Here's how the part is built. I have some questions about the finished solid (model axes, mm). Face numbers are marked on the shaded views. A direction names the side the tool comes from. Coordinates: 2 decimals unless noted, no trailing zeros. Write each loop counter-clockwise with the first axis right and the second up, starting at its lowest first coordinate (ties: lowest second). Pieces come first, ordered by that corner, then holes.
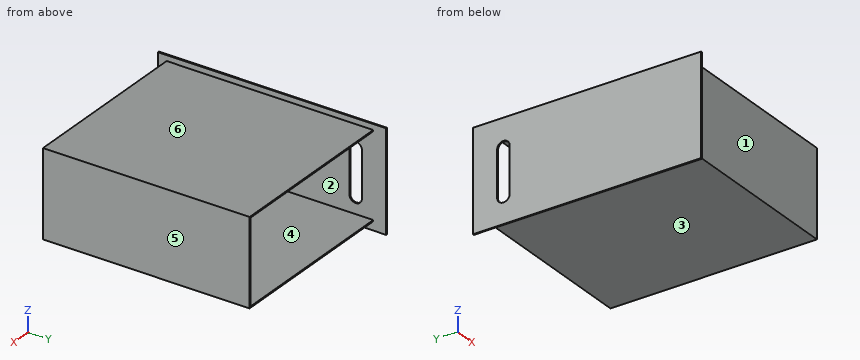
```python
from build123d import *

# Parameters (mm, degrees)
SKETCH_1_W          = 420
SKETCH_1_H          = 200
EXTRUDE_1_DEPTH     = 3
SKETCH_2_W          = 420
SKETCH_2_H          = 200
SKETCH_2_W_2        = 414
SKETCH_2_H_2        = 194
EXTRUDE_1_2_DEPTH   = 477
SKETCH_4_W          = 233
SKETCH_4_H          = 530
EXTRUDE_2_DEPTH     = 3
CUT_EXTRUDE_1_DEPTH = 3


with BuildPart() as part:
    # 草图1 → Extrude 1 (new body)
    with BuildSketch(Plane(origin=(0, 0, 0), x_dir=(1, 0, 0), z_dir=(0, 1, 0))):
        Rectangle(SKETCH_1_W, SKETCH_1_H)
    extrude(amount=EXTRUDE_1_DEPTH)

    # 草图2 → Extrude 1 2 (add)
    with BuildSketch(Plane(origin=(0, 3, 0), x_dir=(1, 0, 0), z_dir=(0, 1, 0))):
        Rectangle(SKETCH_2_W, SKETCH_2_H)
        Rectangle(SKETCH_2_W_2, SKETCH_2_H_2, mode=Mode.SUBTRACT)
    extrude(amount=EXTRUDE_1_2_DEPTH)

    # 草图4 → 凸台-拉伸2 (add)
    with BuildSketch(Plane.ZY.offset(210)):
        with Locations((-3.5, 245)):
            Rectangle(SKETCH_4_W, SKETCH_4_H)
    extrude(amount=-EXTRUDE_2_DEPTH)

    # 草图5 → 切除-拉伸1 (cut)
    with BuildSketch(Plane.ZY.offset(210)):
        with BuildLine():
            Line((-58.054561009, 453.925202317), (47.32277396, 453.925202317))
            ThreePointArc((47.32277396, 453.925202317), (61.958514928, 439.289461349), (47.32277396, 424.653720381))
            Line((47.32277396, 424.653720381), (-58.054561009, 424.653720381))
            ThreePointArc((-58.054561009, 424.653720381), (-72.690301977, 439.289461349), (-58.054561009, 453.925202317))
        make_face()
    extrude(amount=-CUT_EXTRUDE_1_DEPTH, mode=Mode.SUBTRACT)


solid = part.part
```
1) Imagine slicing it at C-C on x = -60. Please give me the cut outline in (y, z), then the cut area to 3 significant figures.
Values follow:
outline: (0, -100) - (480, -100) - (480, -97) - (3, -97) - (3, 97) - (480, 97) - (480, 100) - (0, 100) - close
area: 3,460 mm2
2) Imagine slicing it at A-A on y = 162. Please give me the cut outline in (x, z), then the cut area to 3 significant figures.
Values follow:
outline: (-210, -120) - (-207, -120) - (-207, -100) - (210, -100) - (210, 100) - (-207, 100) - (-207, 113) - (-210, 113) - close; hole (-207, -97) - (207, -97) - (207, 97) - (-207, 97) - close
area: 3,780 mm2
3) Imagine slicing it at D-D on z = -91. Please give me the cut outline in (x, y), then the cut area to 3 significant figures.
Values follow:
outline: (-210, -20) - (-207, -20) - (-207, 0) - (210, 0) - (210, 480) - (207, 480) - (207, 3) - (-207, 3) - (-207, 510) - (-210, 510) - close
area: 4,270 mm2
4) On a 3-axis mill with a long thin cutter (end or side, diameter ignored), from which of +Z, -Z, +X, -X, +Y, -Y can I reach the whole of each face in a straight line? I mean the marked faces 5 and 6. Say none if no direction works.
Values follow:
face 5: +Z, -Z, +X, +Y, -Y
face 6: +Z, +X, +Y, -Y
5) Will these pins go through, and if not, where does the flat tip stop? pin 1 (6 mm diameter, centred on x = 64.5, z = -61, fed in from +Y); pin 2 (2 mm diameter, centred on x = 164, y = 172, fed in from -Z); pin 3 (8 mm diameter, centred on x = 17, z = 17.5, fed in from -Y).
Values follow:
pin 1: stops at y = 3
pin 2: stops at z = -100
pin 3: stops at y = 0
6) I need wall thicknesses on probe 1 along X at (y, z) = (320, -42.5); probe 2 along Z at (x, y) = (-73.5, 472.5); probe 3 along Y at (x, z) = (-130, -86). Which ranges of each line are inside material? Lowest first, please.
Values follow:
probe 1: x = -210 to -207, 207 to 210
probe 2: z = -100 to -97, 97 to 100
probe 3: y = 0 to 3
7) We'd pull the mould along Z, two halves only. Please class the marked faces 1, 2, 3 and 4: pulls with the +Z half, pulls with the -Z half, needs draft (parallel to the pull), parting line crosses it, or undercut.
Values follow:
face 1: needs draft
face 2: undercut
face 3: pulls with the -Z half
face 4: undercut
8) Imagine slicing it at B-B on z = 26. Please give me the cut outline in (x, y), then the cut area to 3 significant figures.
Values follow:
outline: (-210, -20) - (-207, -20) - (-207, 0) - (210, 0) - (210, 480) - (207, 480) - (207, 3) - (-207, 3) - (-207, 424.65) - (-210, 424.65) - close; (-210, 453.93) - (-207, 453.93) - (-207, 510) - (-210, 510) - close
area: 4,180 mm2
